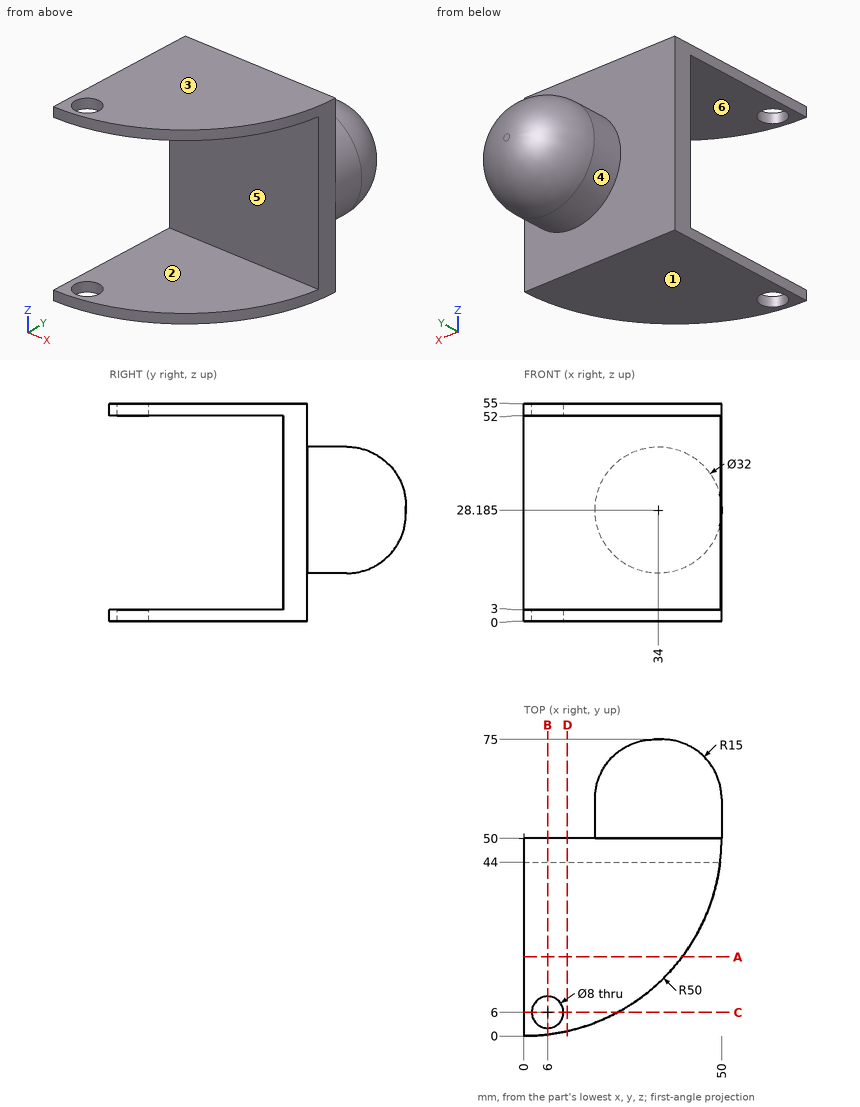
Job drawing, mm, ordinate dimensions from the low corner. One solid piece. A direction names the side the tool comes from. Coordinates: 2 decimals unless noted, no trailing zeros. Write each loop counter-clockwise with the first axis right and the second up, starting at its lowest first coordinate (ties: lowest second). Pieces come first, ordered by that corner, then holes. Notation, with made-up numbers: (55.25, 14) - (113.25, 14) arc R18 ccw to (113.25, 40) - close; hole circle Ø9 at (86, 63.5). An arc over 180 degrees is marked (long way). Use a Markdown table: item, result. Add a question column.
Item 1: Band-saw the part on C-C, the plane y = 6. Give the cut face in (x, z).
Item 2: Mould opens along Z. For the marked faces 3, 4, 5 and 6 say: pulls with the +Z half, pulls with the -Z half, needs draft (parallel to the pull), parting line crosses it, or undercut.
Item 3: Drill centre lines: L1, parallel to Z at x = 24, y = 30.5; L2, parallel to Y at x = 30, z = 49.5; L3, parallel to Y at x = 6, z = 54. Where is each one in solid material? Low to high. Write a range as from..to.
Item 4: Flat gauge pins, fed straight in: pin 1 (2 mm diameter, centred on x = 16.5, z = 49.5, fed in from -Y); pin 2 (6.5 mm diameter, centred on x = 6, y = 6, fed in from +Z); pin 3 (6 mm diameter, centred on y = 44.5, z = 43, fed in from +X); pin 4 (1.5 mm diameter, centred on x = 10.5, z = 44, fed in from +Y). Where does each tip first touch, or does it go through?
Item 5: Band-saw the part on B-B, the plane x = 6. Give the cut face in (y, z).
Item 6: 3-axis set-ups, long thin cutter, end or side, ignore diameter. For the marked faces 1 and 2: which of +Z, -Z, +X, -X, +Y, -Y reach the whole face in a straight line?
Item 7: Band-saw the part on D-D, the plane x = 11. Give the cut face in (y, z) (1 decimal).
Item 8: Band-saw the part on A-A, the plane y = 20. Give the cut face in (x, z), and give its area (3 significant figures).
Numbers:
| question | item | result |
|---|---|---|
| 1 | outline | (0, 0) - (2, 0) - (2, 3) - (0, 3) - close; (0, 52) - (2, 52) - (2, 55) - (0, 55) - close; (10, 0) - (23.75, 0) - (23.75, 3) - (10, 3) - close; (10, 52) - (23.75, 52) - (23.75, 55) - (10, 55) - close |
| 2 | face 3 | pulls with the +Z half |
| 2 | face 4 | parting line crosses it |
| 2 | face 5 | undercut |
| 2 | face 6 | undercut |
| 3 | L1 | 0..3, 52..55 |
| 3 | L2 | 44..50 |
| 3 | L3 | 0.36..2, 10..50 |
| 4 | pin 1 | y = 44 |
| 4 | pin 2 | through |
| 4 | pin 3 | x = 49.94 |
| 4 | pin 4 | y = 50 |
| 5 | outline | (0.36, 0) - (2, 0) - (2, 3) - (0.36, 3) - close; (0.36, 52) - (2, 52) - (2, 55) - (0.36, 55) - close; (10, 0) - (50, 0) - (50, 55) - (10, 55) - (10, 52) - (44, 52) - (44, 3) - (10, 3) - close |
| 6 | face 1 | -Z, +X, -X, +Y, -Y |
| 6 | face 2 | +X, -X, -Y |
| 7 | outline | (1.2, 0) - (50, 0) - (50, 55) - (1.2, 55) - (1.2, 52) - (44, 52) - (44, 3) - (1.2, 3) - close |
| 8 | outline | (0, 0) - (40, 0) - (40, 3) - (0, 3) - close; (0, 52) - (40, 52) - (40, 55) - (0, 55) - close |
| 8 | area | 240 mm2 |
